Answer from the drawing. Dimensions are ordinates in mm from the lowest x, y and z of the part. A direction names the side the tool comes from. Coordinates: 2 decimals unless noted, no trailing zeros. Write each loop counter-clockwise with the first axis right and the second up, starting at its lowest first coordinate (ties: lowest second). Pieces come first, ordered by that corner, then holes. Notation, with made-up numbers: (72.25, 30) - (81.25, 30) arc R21 ccw to (81.25, 44) - close; hole circle Ø11 at (64.5, 30). An arc over 180 degrees is marked (long way). Return JSON: item names as keys, results as strings.
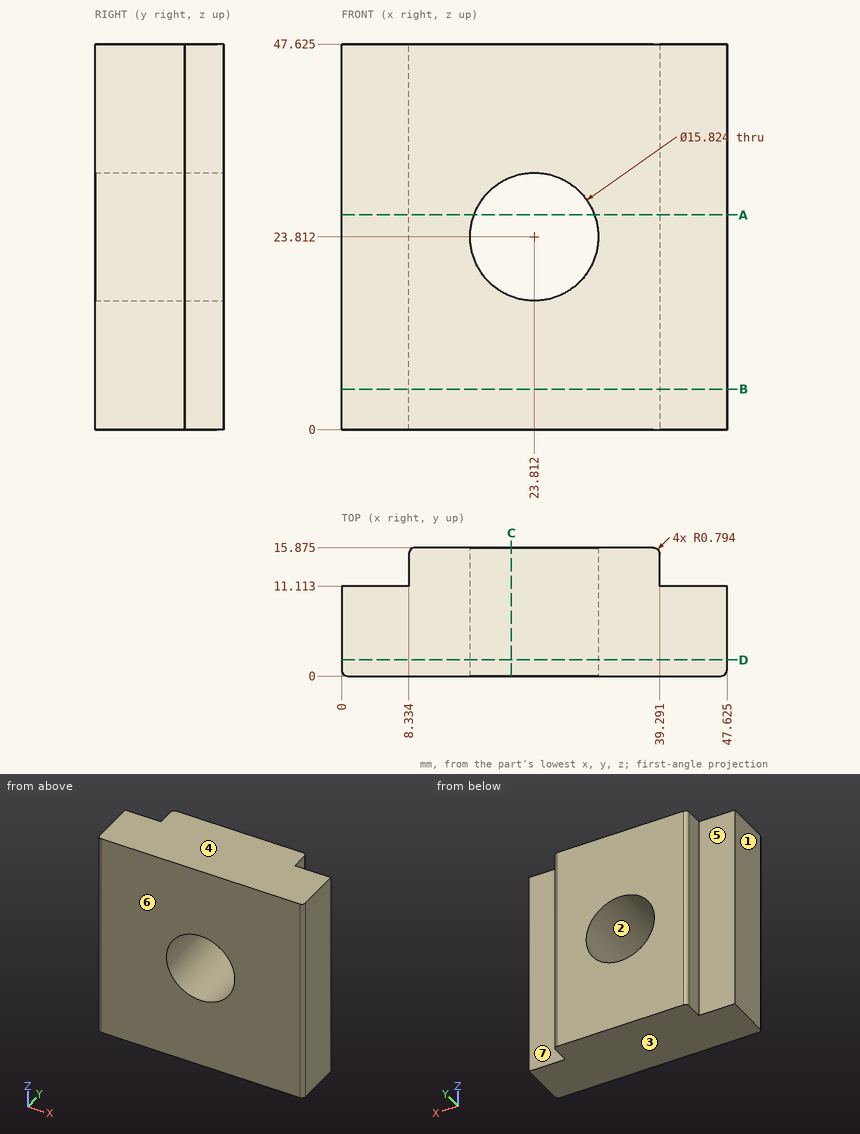
(1) Flat-ended cylindrical pins translate along their axes: P1, Ø6.5, axis at x = 2.5, z = 21, coming from the +Y side; P2, Ø1.2, axis at y = 12.5, z = 33, coming from the -X side; P3, Ø1.5, axis at y = 12, z = 17, coming from the +X side; P4, Ø5, axis at y = 4, z = 22, coming from the -X side. Find the tip coordinate at first contact, or state that the pin passes through.
Answer:
{"P1": "y = 11.11", "P2": "x = 8.33", "P3": "x = 39.29", "P4": "x = 0"}
(2) A cutting plane is placed at B-B (z = 5). Determine the outline of the cut face in (x, y) (1 decimal).
Answer:
{"outline": "(0, 0.8) arc R0.8 ccw to (0.8, 0) - (46.8, 0) arc R0.8 ccw to (47.6, 0.8) - (47.6, 11.1) - (39.3, 11.1) - (39.3, 15.1) arc R0.8 ccw to (38.5, 15.9) - (9.1, 15.9) arc R0.8 ccw to (8.3, 15.1) - (8.3, 11.1) - (0, 11.1) - close"}
(3) A cutting plane is placed at A-A (z = 26.5). Determine the outline of the cut face in (x, y) (1 decimal).
Answer:
{"outline": "(0, 0.8) arc R0.8 ccw to (0.8, 0) - (16.4, 0) - (16.4, 15.9) - (9.1, 15.9) arc R0.8 ccw to (8.3, 15.1) - (8.3, 11.1) - (0, 11.1) - close; (31.3, 0) - (46.8, 0) arc R0.8 ccw to (47.6, 0.8) - (47.6, 11.1) - (39.3, 11.1) - (39.3, 15.1) arc R0.8 ccw to (38.5, 15.9) - (31.3, 15.9) - close"}
(4) Which of the six approach directions +Z, -Z, +X, -X, +Y, -Y give full straight-line access (tool end or side, diameter ignored) to the marked faces 5, 6 and 7?
Answer:
{"face 5": "+Z, -Z, -X, +Y", "face 6": "+Z, -Z, +X, -X, -Y", "face 7": "+Z, -Z, +X, +Y"}
(5) A cutting plane is placed at D-D (y = 2). Determine the outline of the cut face in (x, z) (1 decimal), and give its area (3 significant figures).
Answer:
{"outline": "(0, 0) - (47.6, 0) - (47.6, 47.6) - (0, 47.6) - close; hole circle Ø15.8 at (23.8, 23.8)", "area": "2,070 mm²"}
(6) Straight lines are drawn through the part: line 1 (Z direction, x = 24, y = 4.5) (1 decimal); line 2 (Y direction, x = 41, z = 29); line 3 (Z direction, x = 16.5, y = 11) (1 decimal). For each, find the intervals that lie inside material, in ascending order. Write a range as from..to.
Answer:
{"line 1": "0..15.9, 31.7..47.6", "line 2": "0..11.11", "line 3": "0..20.8, 26.8..47.6"}
(7) A cutting plane is placed at C-C (x = 21). Determine the outline of the cut face in (y, z) (1 decimal).
Answer:
{"outline": "(0, 0) - (15.9, 0) - (15.9, 16.4) - (0, 16.4) - close; (0, 31.2) - (15.9, 31.2) - (15.9, 47.6) - (0, 47.6) - close"}
(8) Determine the mould class of the marked faces 1, 2, 3 and 4 for opening direction Z: +Z half, -Z half, draft (parallel to the pull), parting line (faces both ways), or undercut.
Answer:
{"face 1": "draft", "face 2": "undercut", "face 3": "-Z half", "face 4": "+Z half"}
